from build123d import *

# Parameters (mm, degrees)
SKETCH_W        = 60
SKETCH_H        = 90
PAD_DEPTH       = 10
SKETCH001_W     = 30
SKETCH001_H     = 60
POCKET_DEPTH    = 10.001
SKETCH002_W     = 36
SKETCH002_H     = 70
POCKET001_DEPTH = 7.5
SKETCH003_R     = 25.5
POCKET002_DEPTH = 5


with BuildPart() as part:
    # Sketch → Pad (new body)
    with BuildSketch(Plane.XY):
        with Locations((30, 45)):
            Rectangle(SKETCH_W, SKETCH_H)
    extrude(amount=PAD_DEPTH)

    # Sketch001 (on Face5 of Pad) → Pocket (cut, through all)
    with BuildSketch(Plane(origin=(0, 0, 0), x_dir=(1, 0, 0), z_dir=(0, 0, -1))):
        with Locations((30, -45)):
            Rectangle(SKETCH001_W, SKETCH001_H)
    extrude(amount=-POCKET_DEPTH, mode=Mode.SUBTRACT)

    # Sketch002 → Pocket001 (cut)
    with BuildSketch(Plane.XY):
        with Locations((30, 45)):
            Rectangle(SKETCH002_W, SKETCH002_H)
    extrude(amount=POCKET001_DEPTH, mode=Mode.SUBTRACT)

    # Sketch003 → Pocket002 (cut)
    with BuildSketch(Plane.XY):
        with Locations((30, 45)):
            Circle(SKETCH003_R)
    extrude(amount=POCKET002_DEPTH, mode=Mode.SUBTRACT)


solid = part.part
Verification items for the finished model (mm, model axes). A direction names the side the tool comes from. Round coordinates to 2 decimals unless told otherwise and drop trailing zeros. Loops run counter-clockwise (first coordinate to the right, second up) from the corner with the lowest first, then second, coordinate; pieces in that order, holes last. Notation, with made-up numbers: (46.25, 46) - (101.25, 46) arc R20 cw to (101.25, 77) - close; hole circle Ø4 at (36, 3). An arc over 180 degrees is marked (long way). Use a Markdown table: item, result. Add a question column.
1. Release check for a two-part mould opening along Y. For faces 4 (the face through (50, 46, 10)), 5 (the face through (30, 0, 5)), 6 (the face through (30, 90, 5)), 7 (the face through (15, 45, 9)) record: released by +Y, released by -Y, zero draft, split by the parting line, or undercut.
2. Section check D-D, the plane x = 46.5. Record the boundary of the cut face in (y, z), plus the area to 3 significant figures.
3. Gauge pin test, flat end, axial feed: pin 1 (4 mm diameter, centred on x = 10, y = 38.5, fed in from -Z). Record the tip position at first contact, or that the pin passes through.
4. Section check C-C, the plane z = 6.5. Record the boundary of the cut face in (x, y).
5. Thickness scan on probe 1 along Y at (x, z) = (42.5, 1.75); probe 2 along X at (y, z) = (74.5, 7); probe 3 along Y at (x, z) = (27.5, 8). Record the ranges inside material, lowest first. Write a range as [from, to].
6. Section check A-A, the plane y = 25. Record the boundary of the cut face in (x, z), plus the area to 3 significant figures.
7. Section check B-B, the plane x = 29. Record the boundary of the cut face in (y, z).
8. Access from +Z, -Z, +X, -X, +Y, -Y to the whole of each face (thin tool, end or side, straight path). Record for faces 1 (the face through (9, 45, 5)), 2 (the face through (30, 15, 9)), 3 (the face through (0, 44, 5)).
Checks:
| question | item | result |
|---|---|---|
| 1 | face 4 | zero draft |
| 1 | face 5 | released by -Y |
| 1 | face 6 | released by +Y |
| 1 | face 7 | undercut |
| 2 | outline | (0, 0) - (10, 0) - (10, 7.5) - (80, 7.5) - (80, 0) - (90, 0) - (90, 10) - (0, 10) - close |
| 2 | area | 375 mm^2 |
| 3 | pin 1 | stops at z = 5 |
| 4 | outline | (0, 0) - (60, 0) - (60, 90) - (0, 90) - close; hole (12, 10) - (48, 10) - (48, 80) - (12, 80) - close |
| 5 | probe 1 | y = [0, 10], [80, 90] |
| 5 | probe 2 | x = [0, 12], [48, 60] |
| 5 | probe 3 | y = [0, 15], [75, 90] |
| 6 | outline | (0, 0) - (12, 0) - (12, 7.5) - (15, 7.5) - (15, 10) - (0, 10) - close; (45, 7.5) - (48, 7.5) - (48, 0) - (60, 0) - (60, 10) - (45, 10) - close |
| 6 | area | 255 mm^2 |
| 7 | outline | (0, 0) - (10, 0) - (10, 7.5) - (15, 7.5) - (15, 10) - (0, 10) - close; (75, 7.5) - (80, 7.5) - (80, 0) - (90, 0) - (90, 10) - (75, 10) - close |
| 8 | face 1 | -Z |
| 8 | face 2 | +Z, -Z |
| 8 | face 3 | +Z, -Z, -X, +Y, -Y |
